Could you check a few things on this model? Use its own coordinates, in mm. Face numbers are marked on the shaded views. A direction names the side the tool comes from. Give positions to 0.01 mm unless a question says otherwise; leave off trailing zeros. Loops run counter-clockwise (first coordinate to the right, second up) from the corner with the lowest first, then second, coordinate; pieces in that order, holes last. Notation, with made-up numbers: M -11.75,52.5 L 4.25,52.5 A20 cw 4.25,71.5 Z; hole C 35,74 d3. An arc over 180 degrees is marked long. Return JSON: item names as keys, results as strings. Group by question number.
1. If we section it at D-D (y = 45.5): Write out the boundary of the cut face in (x, z), plus the area to 3 significant figures.
2. For the marked faces 1, 2 and 3, which set-ups out of +Z, -Z, +X, -X, +Y, -Y let a thin tool reach every point of the face, with its end or its side?
3. For pin 1 (10 mm diameter, centred on x = -13.5, z = -1.5, fed in from -Y); pin 2 (8 mm diameter, centred on y = 82.5, z = -11.5, fed in from +X); pin 3 (12 mm diameter, centred on x = -4, y = 63.5, fed in from -Z); pin 4 (1.5 mm diameter, centred on x = -7, y = 42, fed in from -Z), each with a flat end and sliding along its axis, tell me the tip position at first contact or that it passes through.
4. If we section it at A-A (y = -9.5): Write out the boundary of the cut face in (x, z), plus the area to 3 significant figures.
5. Please list where these lines run through material, in increasing order: line 1 (Y direction, x = -17.5, z = -11) (3 decimals); line 2 (Y direction, x = -7, z = -16.5) (3 decimals); line 3 (Z direction, x = -1, y = 94.5).
6. If we section it at B-B (x = 8.5): Write out the boundary of the cut face in (y, z) (3 decimals), plus the area to 3 significant figures.
7. If we section it at C-C (x = -11.5): Write out the boundary of the cut face in (y, z) (3 decimals), plus the area to 3 significant figures.
```python
from build123d import *

# Parameters (mm, degrees)
SKETCH1_W           = 38.1
SKETCH1_H           = 38.1
SKETCH1_R           = 1.499997
BOSS_EXTRUDE1_DEPTH = 4.445
SKETCH2_R           = 19.05
BOSS_EXTRUDE2_DEPTH = 114.3
SKETCH3_R           = 4
BOSS_EXTRUDE3_DEPTH = 25.4


with BuildPart() as part:
    # Sketch1 → Boss-Extrude1 (new body)
    with BuildSketch(Plane(origin=(0, 0, 0), x_dir=(1, 0, 0), z_dir=(0, 1, 0))):
        Rectangle(SKETCH1_W, SKETCH1_H)
        with Locations(Location((-16.050006, 16.050006, 0), (0, 0, 270))):
            Circle(SKETCH1_R, mode=Mode.SUBTRACT)
        with Locations(Location((16.050006, 16.050006, 0), (0, 0, 90))):
            Circle(SKETCH1_R, mode=Mode.SUBTRACT)
        with Locations(Location((16.050006, -16.050006, 0), (0, 0, 270))):
            Circle(SKETCH1_R, mode=Mode.SUBTRACT)
        with Locations(Location((-16.050006, -16.050006, 0), (0, 0, 90))):
            Circle(SKETCH1_R, mode=Mode.SUBTRACT)
    extrude(amount=BOSS_EXTRUDE1_DEPTH)

    # Sketch2 → Boss-Extrude2 (add)
    with BuildSketch(Plane(origin=(0, 4.445, 0), x_dir=(1, 0, 0), z_dir=(0, 1, 0))):
        with Locations(Location((0, 0, 0), (0, 0, 270))):
            Circle(SKETCH2_R)
    extrude(amount=BOSS_EXTRUDE2_DEPTH)

    # Sketch3 → Boss-Extrude3 (add)
    with BuildSketch(Plane.XZ):
        with Locations(Location((0, 0, 0), (0, 0, 270))):
            Circle(SKETCH3_R)
    extrude(amount=BOSS_EXTRUDE3_DEPTH)


solid = part.part
```
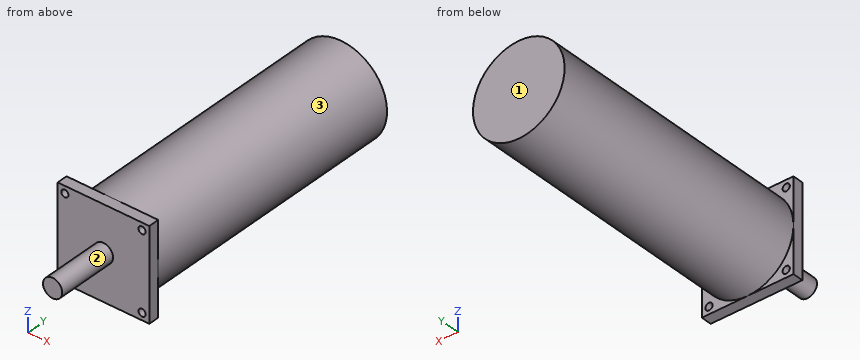
Answer:
{
 "1": {"outline": "C 0,0 d38.1", "area": "1,140 mm²"},
 "2": {"face 1": "+Z, -Z, +X, -X, +Y", "face 2": "-Y", "face 3": "+Y"},
 "3": {"pin 1": "stops at y = 0", "pin 2": "stops at x = 17.51", "pin 3": "stops at z = -19.05", "pin 4": "stops at z = -18"},
 "4": {"outline": "C 0,0 d8", "area": "50.3 mm²"},
 "5": {"line 1": "y = 0 to 4.445", "line 2": "y = 0 to 118.745", "line 3": "z = -19.02 to 19.02"},
 "6": {"outline": "M 0,-19.05 L 4.445,-19.05 L 4.445,-17.049 L 118.745,-17.049 L 118.745,17.049 L 4.445,17.049 L 4.445,19.05 L 0,19.05 Z", "area": "4,070 mm²"},
 "7": {"outline": "M 0,-19.05 L 4.445,-19.05 L 4.445,-15.187 L 118.745,-15.187 L 118.745,15.187 L 4.445,15.187 L 4.445,19.05 L 0,19.05 Z", "area": "3,640 mm²"}
}
